from build123d import *

# Parameters (mm, degrees)
SKETCH1_W                  = 38.1
SKETCH1_H                  = 50.8
BOSS_EXTRUDE1_DEPTH        = 31.75
SKETCH2_R                  = 11.1125
CUT_EXTRUDE1_DEPTH         = 45.901280605
SKETCH3_W                  = 28.575
SKETCH3_H                  = 9.525
CUT_EXTRUDE2_DEPTH         = 45.901280605
F_10_CLEARANCE_HOLE1_D     = 5.1054
F_10_CLEARANCE_HOLE1_DEPTH = 9.652
F_10_CLEARANCE_HOLE1_TIP   = 1.533816902
SKETCH6_W                  = 3.175
SKETCH6_H                  = 31.75
CUT_EXTRUDE3_DEPTH         = 24.13
F_10_CLEARANCE_HOLE2_D     = 5.1054


with BuildPart() as part:
    # Sketch1 → Boss-Extrude1 (new body)
    with BuildSketch(Plane(origin=(0, 0, 0), x_dir=(1, 0, 0), z_dir=(0, 1, 0))):
        Rectangle(SKETCH1_W, SKETCH1_H)
    extrude(amount=BOSS_EXTRUDE1_DEPTH)

    # Sketch2 → Cut-Extrude1 (cut, through all)
    with BuildSketch(Plane(origin=(0, 31.75, 0), x_dir=(1, 0, 0), z_dir=(0, 1, 0))):
        with Locations(Location((-3.175, 0, 0), (0, 0, 270))):
            Circle(SKETCH2_R)
    extrude(amount=-CUT_EXTRUDE1_DEPTH, mode=Mode.SUBTRACT)

    # Sketch3 → Cut-Extrude2 (cut, through all)
    with BuildSketch(Plane(origin=(0, 31.75, 0), x_dir=(1, 0, 0), z_dir=(0, 1, 0))):
        with Locations((4.7625, 20.6375)):
            Rectangle(SKETCH3_W, SKETCH3_H)
        with Locations((4.7625, -20.6375)):
            Rectangle(SKETCH3_W, SKETCH3_H)
    extrude(amount=-CUT_EXTRUDE2_DEPTH, mode=Mode.SUBTRACT)

    # #10 Clearance Hole1
    with Locations(Plane(origin=(-9.525, 0, 0), x_dir=(0, 0, -1), z_dir=(1, 0, 0))):
        with Locations((-20.6375, 25.4), (20.6375, 6.35), (-20.6375, 6.35), (20.6375, 25.4)):
            Hole(F_10_CLEARANCE_HOLE1_D / 2, depth=F_10_CLEARANCE_HOLE1_DEPTH)
            with Locations((0, 0, -(F_10_CLEARANCE_HOLE1_DEPTH + F_10_CLEARANCE_HOLE1_TIP / 2))):  # 118° drill point
                Cone(0, F_10_CLEARANCE_HOLE1_D / 2, F_10_CLEARANCE_HOLE1_TIP, mode=Mode.SUBTRACT)

    # Sketch6 → Cut-Extrude3 (cut)
    with BuildSketch(Plane(origin=(19.05, 0, 0), x_dir=(0, 0, -1), z_dir=(1, 0, 0))):
        with Locations((0, 15.875)):
            Rectangle(SKETCH6_W, SKETCH6_H)
    extrude(amount=-CUT_EXTRUDE3_DEPTH, mode=Mode.SUBTRACT)

    # #10 Clearance Hole2 (through all)
    with Locations(Plane.XY.offset(15.875)):
        with Locations((12.7, 15.875)):
            Hole(F_10_CLEARANCE_HOLE2_D / 2)


solid = part.part
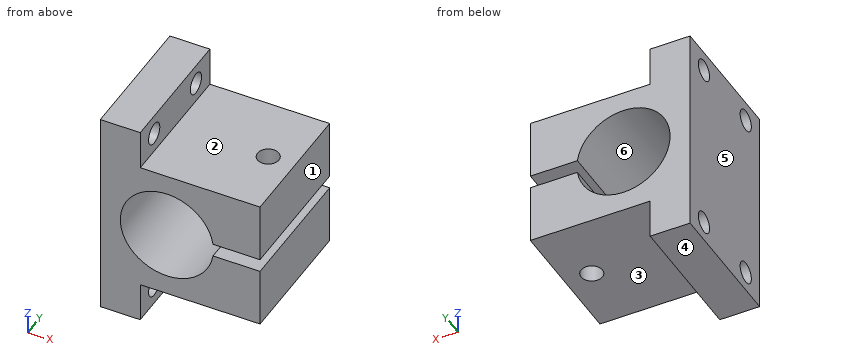
Check sheet for the modelled part. Datum: model origin and axes. Units: mm. Face numbers are marked on the shaded views. A direction names the side the tool comes from. Round coordinates to 2 decimals unless told otherwise and drop trailing zeros. Order: outer loops, then holes, each group sorted by start corner. A loop starts at its lowest first (then second) coordinate and runs counter-clockwise, first axis right, second up. Notation, with made-up numbers: M -29,32 L -14,32 A20 cw -14,70 Z; hole C -17.5,-26.75 d1. An arc over 180 degrees is marked long. One line per item, written item: value. Start each with the question number.
1. Scan lines: line 1 along Z through (x, y) = (-15, 25); line 2 along Y through (x, z) = (12.5, 8.5); line 3 along Y through (x, z) = (-17, -18.5). Record each from-to range of solid material in increasing order.
2. Section check D-D on z = 12. Enter the section's corners in (x, y) (3 decimals).
3. Section check C-C on z = 6. Enter the section's corners in (x, y) (3 decimals).
4. Gauge pin test, flat ends, axial feed: P1, Ø14.5, axis at x = 8.5, y = 18, coming from the +Z side (3 decimals); P2, Ø14.5, axis at x = 2, y = 18, coming from the -Z side (3 decimals); P3, Ø3, axis at y = 21.5, z = -18.5, coming from the +X side (3 decimals). Record the tip position at first contact, or that the pin passes through.
5. Release check for a two-part mould opening along X. For the marked faces 4, 5 and 6 record: released by +X, released by -X, zero draft, split by the parting line, or undercut.
6. Access from +Z, -Z, +X, -X, +Y, -Y to the whole of each face (thin tool, end or side, straight path). Record for the marked faces 1, 2 and 3.
7. Section check A-A on y = 25.4. Give the number of separate pieces and of enclosed holes in the cut face, and give its area (3 significant figures).
Results found:
1. line 1: -25.4 to -23.16, -18.12 to 18.12, 23.16 to 25.4
1. line 2: 0 to 13.33, 18.42 to 31.75
1. line 3: 0 to 4.95, 7.75 to 24, 26.8 to 31.75
2. outline: M -19.05,0 L 19.05,0 L 19.05,31.75 L -19.05,31.75 Z; hole C 12.7,15.875 d5.105
3. outline: M -19.05,0 L -12.528,0 L -12.528,31.75 L -19.05,31.75 Z; M 6.178,0 L 19.05,0 L 19.05,31.75 L 6.178,31.75 Z; hole C 12.7,15.875 d5.105
4. P1: z = 15.875
4. P2: z = -15.875
4. P3: x = -9.525
5. face 4: zero draft
5. face 5: released by -X
5. face 6: undercut
6. face 1: +Z, -Z, +X, +Y, -Y
6. face 2: +Z, +X, +Y, -Y
6. face 3: -Z, +X, +Y, -Y
7. separate pieces: 3
7. enclosed holes: 0
7. area: 871 mm^2
